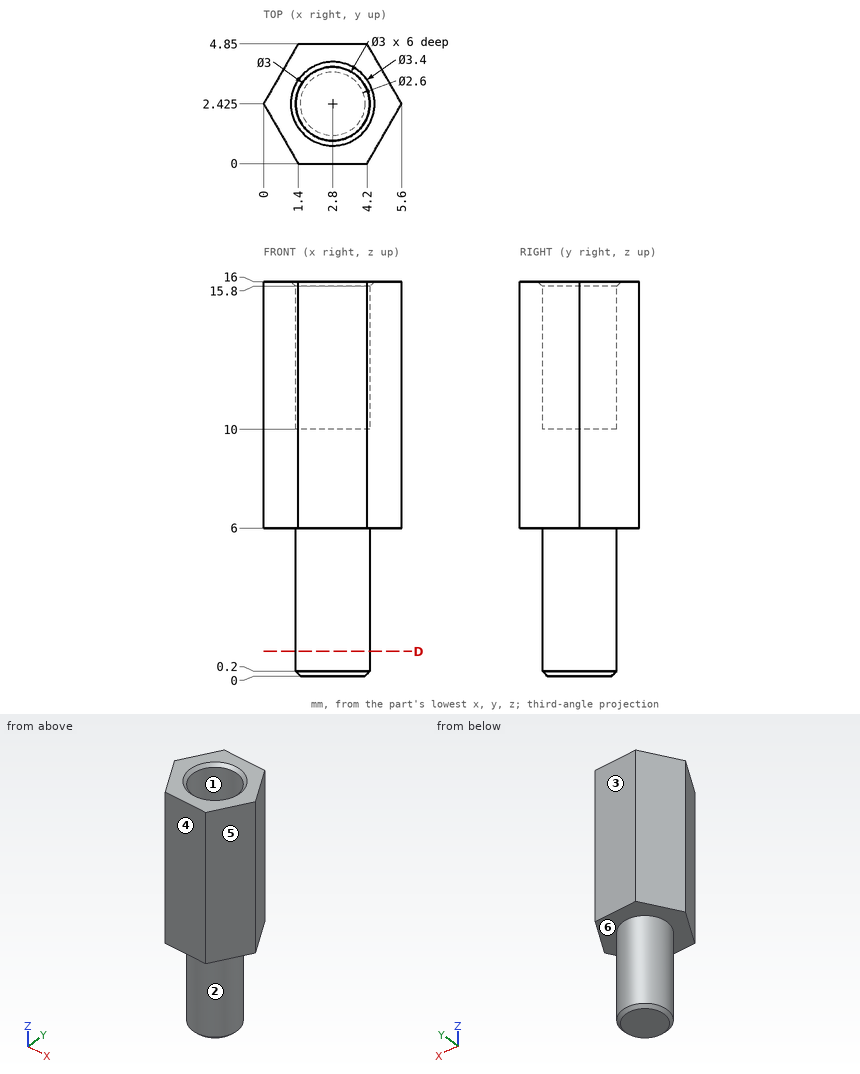
Source: three-view drawing plus pictorial views. Frame: mm from the lowest corner of the part. A direction names the side the tool comes from. Round coordinates to 2 decimals unless told otherwise and drop trailing zeros. Order: outer loops, then holes, each group sorted by start corner. A loop starts at its lowest first (then second) coordinate and runs counter-clockwise, first axis right, second up. Notation, with made-up numbers: (41, 78) - (48, 78) arc R16 ccw to (48, 100) - close; hole circle Ø7 at (44, -22.5). An arc over 180 degrees is marked (long way). Use a Markdown table: item, result.
1. Mould query, pull axis Y, two halves, no side actions, for the marked faces 1, 2, 3 and 4. Classes: +Y half, -Y half, draft (parallel to the pull), parting line (faces both ways), or undercut.
Evaluation:
| item | result |
|---|---|
| face 1 | undercut |
| face 2 | parting line |
| face 3 | +Y half |
| face 4 | -Y half |
2. Material intervals for probe 1 along Z at (x, y) = (0.6, 1.8); probe 2 along X at (y, z) = (3.6, 14.25); probe 3 along X at (y, z) = (2.8, 13.25), sorted ascending.
Evaluation:
| item | result |
|---|---|
| probe 1 | 6 to 16 |
| probe 2 | 0.68 to 1.87, 3.73 to 4.92 |
| probe 3 | 0.22 to 1.35, 4.25 to 5.38 |
3. Access query for the marked faces 5 and 6. Directions: +Z, -Z, +X, -X, +Y, -Y. A direction counts if a zero-diameter tool reaches every point of the face in a straight line with its end or side. Return the directions, or none.
Evaluation:
| item | result |
|---|---|
| face 5 | +Z, -Z, +X, -Y |
| face 6 | -Z |
4. Section D-D on z = 1. Return the cut outline in (x, y) (1 decimal).
Evaluation:
| item | result |
|---|---|
| outline | circle Ø3 at (2.8, 2.4) |
5. First-contact query: pin 1 (1.5 mm diameter, centred on y = 1, z = 8, fed in from -X); pin 2 (1.5 mm diameter, centred on x = 2.5, y = 2, fed in from +Z); pin 3 (2 mm diameter, centred on x = 1, z = 4.5, fed in from +Y). Flat tips, straight axial feed; report the tip coordinate or a pass-through.
Evaluation:
| item | result |
|---|---|
| pin 1 | x = 0.39 |
| pin 2 | z = 10 |
| pin 3 | y = 3.69 |
